Job drawing, mm, ordinate dimensions from the low corner. One solid piece. A direction names the side the tool comes from. Round coordinates to 2 decimals unless told otherwise and drop trailing zeros. Order: outer loops, then holes, each group sorted by start corner. A loop starts at its lowest first (then second) coordinate and runs counter-clockwise, first axis right, second up. Notation, with made-up numbers: (31.25, 72.25) -> (49.25, 72.25) arc R19 cw to (49.25, 100.25) -> close; hole circle Ø7 at (89.25, -2.75). An arc over 180 degrees is marked (long way). Use CSV: the item, a comma, the result in double quotes.
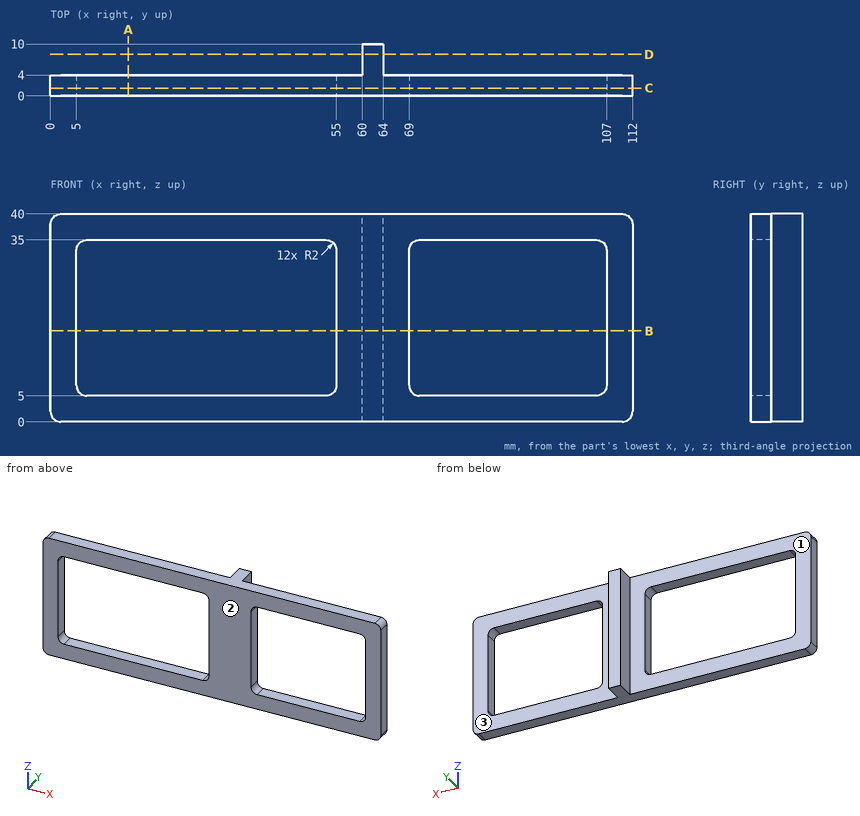
(1) Cut at D-D, the plane y = 8. Give the cut face in (x, z), then the cut area to 3 significant figures.
Reply:
outline,"(60, 0) -> (64, 0) -> (64, 40) -> (60, 40) -> close"
area,"160 mm2"
(2) Cut at C-C, the plane y = 1.5. Give the cut face in (x, z), then the cut area to 3 significant figures.
Reply:
outline,"(0, 2) arc R2 ccw to (2, 0) -> (110, 0) arc R2 ccw to (112, 2) -> (112, 38) arc R2 ccw to (110, 40) -> (2, 40) arc R2 ccw to (0, 38) -> close; hole (5, 7) arc R2 ccw to (7, 5) -> (53, 5) arc R2 ccw to (55, 7) -> (55, 33) arc R2 ccw to (53, 35) -> (7, 35) arc R2 ccw to (5, 33) -> close; hole (69, 7) arc R2 ccw to (71, 5) -> (105, 5) arc R2 ccw to (107, 7) -> (107, 33) arc R2 ccw to (105, 35) -> (71, 35) arc R2 ccw to (69, 33) -> close"
area,"1,840 mm2"
(3) Drop flat-ended pins along their axis: P1, Ø4, axis at y = 7.5, z = 19, coming from the +X side; P2, Ø4, axis at x = 72.5, z = 24, coming from the +Y side; P3, Ø4.5, axis at y = 1.5, z = 16.5, coming from the -X side. Give the stop position or say it passes through.
Reply:
P1,"x = 64"
P2,"through"
P3,"x = 0"
(4) Which spindle directions (+Z, -Z, +X, -X, +Y, -Y) get a long thin tool onto all of the face, cutting with end or side? Do the marked faces 1, 2 and 3. Say none if no direction does.
Reply:
face 1,"+Z, -Z, -X, +Y"
face 2,"+Z, -Z, +X, -X, -Y"
face 3,"+Z, -Z, +X, +Y"
(5) Cut at A-A, the plane x = 15. Give the cut face in (y, z), then the cut area to 3 significant figures.
Reply:
outline,"(0, 0) -> (4, 0) -> (4, 5) -> (0, 5) -> close; (0, 35) -> (4, 35) -> (4, 40) -> (0, 40) -> close"
area,"40.0 mm2"
(6) Probe probe 1 along X at (y, z) = (2, 14); probe 2 along Z at (x, y) = (40.5, 2); probe 3 along X at (y, z) = (7.75, 10). List the from-to ranges inside material, lowest first. Write a range as [from, to].
Reply:
probe 1,"[0, 5], [55, 69], [107, 112]"
probe 2,"[0, 5], [35, 40]"
probe 3,"[60, 64]"
(7) Cut at B-B, the plane z = 17.5. Give the cut face in (x, y), then the cut area to 3 significant figures.
Reply:
outline,"(0, 0) -> (5, 0) -> (5, 4) -> (0, 4) -> close; (55, 0) -> (69, 0) -> (69, 4) -> (64, 4) -> (64, 10) -> (60, 10) -> (60, 4) -> (55, 4) -> close; (107, 0) -> (112, 0) -> (112, 4) -> (107, 4) -> close"
area,"120 mm2"
